from build123d import *

# Parameters (mm, degrees)
SZKIC1_R                         = 11.955497861
SZKIC1_R_2                       = 8
DODANIE_WYCI_GNI_CIE1_DEPTH      = 10
SZKIC2_W                         = 10
SZKIC2_H                         = 23.910995722
DODANIE_WYCI_GNI_CIE2_DEPTH      = 21
SFAZOWANIE1_SIZE                 = 15
SZKIC4_W                         = 9.112824073
SZKIC4_H                         = 13.669236109
DODANIE_WYCI_GNI_CIE4_DEPTH      = 33
DODANIE_WYCI_GNI_CIE5_DEPTH      = 10
DODANIE_WYCI_GNI_CIE5_DEPTH_BACK = 12
SZKIC5_W                         = 41.411530905
SZKIC5_H                         = 13.669236109
SZKIC6_W                         = 16.08298615
SZKIC6_H                         = 27.20632334
WYTNIJ_WYCI_GNI_CIE1_DEPTH       = 54.798638821
WYTNIJ_WYCI_GNI_CIE2_DEPTH       = 54.798638821


with BuildPart() as part:
    # Szkic1 → Dodanie-wyciągnięcie1 (new body)
    with BuildSketch(Plane(origin=(0, 0, 0), x_dir=(0, 0, -1), z_dir=(1, 0, 0))):
        Circle(SZKIC1_R)
        Circle(SZKIC1_R_2, mode=Mode.SUBTRACT)
    extrude(amount=DODANIE_WYCI_GNI_CIE1_DEPTH)

    # Szkic2 → Dodanie-wyciągnięcie2 (add)
    with BuildSketch(Plane.XY):
        with Locations((5, 0)):
            Rectangle(SZKIC2_W, SZKIC2_H)
    extrude(amount=DODANIE_WYCI_GNI_CIE2_DEPTH)

    # Sfazowanie1
    # the kernel refuses this chamfer: 15 mm, written as the material it takes off along each edge
    with BuildSketch(Plane(origin=(0, -50.53074268, 21), x_dir=(0.9996219169112968, 0, 0.02749587661058632), z_dir=(0, 1, 0))) as sfazowanie1_piece_1:
        Polygon((SFAZOWANIE1_SIZE * 0.999621916911, SFAZOWANIE1_SIZE * 0.0274958766106), (-SFAZOWANIE1_SIZE * 0.0274958766106, SFAZOWANIE1_SIZE * 0.999621916911), (0, 0), align=None)
    extrude(amount=101.06148536, mode=Mode.SUBTRACT)

    # Szkic4 → Dodanie-wyciągnięcie4 (add)
    with BuildSketch(Plane(origin=(-3, 0, 3), x_dir=(0.7071067811865513, 0, 0.7071067811865438), z_dir=(-0.7071067811865438, 0, 0.7071067811865513))):
        with Locations((11.369948619, -0.23897266)):
            Rectangle(SZKIC4_W, SZKIC4_H)
    extrude(amount=DODANIE_WYCI_GNI_CIE4_DEPTH)

    # Szkic5 → Dodanie-wyciągnięcie5 (add, two sides: drawn at the far end of the back side and taken through both)
    with BuildSketch(Plane(origin=(11.261637619, 0, 11.261637619), x_dir=(0.7071067811865438, 0, -0.7071067811865512), z_dir=(0.7071067811865512, 0, 0.7071067811865438)).offset(-DODANIE_WYCI_GNI_CIE5_DEPTH_BACK)):
        with Locations((-16.536875235, -0.23897266)):
            Rectangle(SZKIC5_W, SZKIC5_H)
    extrude(amount=DODANIE_WYCI_GNI_CIE5_DEPTH + DODANIE_WYCI_GNI_CIE5_DEPTH_BACK)

    # Szkic6 → Wytnij-wyciągnięcie1 (cut, through all)
    with BuildSketch(Plane(origin=(0, 6.595645395, 0), x_dir=(1, 0, 0), z_dir=(0, 1, 0))):
        with Locations((18.041493075, -17.707460584)):
            Rectangle(SZKIC6_W, SZKIC6_H)
    extrude(amount=-WYTNIJ_WYCI_GNI_CIE1_DEPTH, mode=Mode.SUBTRACT)

    # Szkic7 → Wytnij-wyciągnięcie2 (cut, through all)
    with BuildSketch(Plane(origin=(0, 6.595645395, 0), x_dir=(1, 0, 0), z_dir=(0, 1, 0))):
        Polygon((-23.770482817, -28.898564741), (9.416159533, -28.898564741), (9.416159533, -47.919361128), (-20.148773981, -47.919361128), align=None)
    extrude(amount=-WYTNIJ_WYCI_GNI_CIE2_DEPTH, mode=Mode.SUBTRACT)


solid = part.part
Model file for the job. Use its own axes, mm. A direction names the side the tool comes from. Coordinates: 2 decimals unless noted, no trailing zeros. Write each loop counter-clockwise with the first axis right and the second up, starting at its lowest first coordinate (ties: lowest second). Pieces come first, ordered by that corner, then holes. Notation, with made-up numbers: (-36, 27) -> (-17, 27) arc R13 cw to (-17, 46) -> close; hole circle Ø8 at (38.5, 22). An arc over 180 degrees is marked (long way). One line per item, written item: value. Start each with the question number.
1) Probe probe 1 along Y at (x, z) = (-17.5, 25); probe 2 along Z at (x, y) = (2, -0.5); probe 3 along Z at (x, y) = (6.5, -2.25). List the from-to ranges inside material, lowest first.
2) Slice it at A-A on y = 0. Write the cut outline in (x, z), then the cut area to 3 significant figures.
3) Slice it at B-B on x = 1.5. Write the cut outline in (y, z).
4) Which spindle directions (+Z, -Z, +X, -X, +Y, -Y) get a long thin tool onto all of the face, cutting with end or side? Do faces 1 (the face through (5, 9, 11)), 2 (the face through (10, 0, 8)), 3 (the face through (-3, -7.074, 21)). Say none if no direction does.
5) Slice it at C-C on y = -3. Write the cut outline in (x, z), then the cut area to 3 significant figures.
6) Flat gauge pins, fed straight in: pin 1 Ø1.5 at (x, z) = (-7, 11) entering from -Y; pin 2 Ø4 at (y, z) = (2, 3) entering from -X; pin 3 Ø18.5 at (x, z) = (-5.5, 21) entering from -Y; pin 4 Ø11.5 at (x, z) = (-7.5, 17) entering from +Y. Where does each tip first touch, or does it go through?
7) Slice it at D-D on z = 8. Write the cut outline in (x, y), then the cut area to 3 significant figures.
8) Pull direction Y, two halves, no side cores. Call faces 4 (the face through (5, 0, 0)), 5 (the face through (5, 0, -8)), 6 (the face through (-3, 6.596, 21)), 7 (the face through (0, 0, 1)): +Y half, -Y half, draft (parallel to the pull), parting line (faces both ways), or undercut.
Answers follow:
1. probe 1: -7.07 to 6.6
1. probe 2: -11.95 to -7.98, 0 to 28.9
1. probe 3: -11.74 to -7.68, 0 to 28.9
2. outline: (-23.35, 28.9) -> (0, 5.55) -> (0, 0) -> (5.55, 0) -> (5.72, -0.17) -> (5.9, 0) -> (10, 0) -> (10, 26.67) -> (7.77, 28.9) -> close; (0, -11.96) -> (10, -11.96) -> (10, -8) -> (0, -8) -> close
2. area: 599 mm2
3. outline: (-11.96, 0) arc R11.96 ccw to (11.96, 0) -> (11.96, 7.5) -> (6.6, 7.5) -> (6.6, 28.9) -> (-7.07, 28.9) -> (-7.07, 7.5) -> (-11.96, 7.5) -> close; hole (-8, 0) arc R8 ccw to (8, 0) -> close
4. face 1: +Z, -X, +Y
4. face 2: +Z, -Z, +X, +Y, -Y
4. face 3: +Z, -X, -Y
5. outline: (-23.35, 28.9) -> (0, 5.55) -> (0, 0) -> (5.55, 0) -> (5.72, -0.17) -> (5.9, 0) -> (10, 0) -> (10, 26.67) -> (7.77, 28.9) -> close; (0, -11.57) -> (10, -11.57) -> (10, -7.42) -> (0, -7.42) -> close
5. area: 601 mm2
6. pin 1: through
6. pin 2: x = 0
6. pin 3: y = -7.07
6. pin 4: y = 6.6
7. outline: (-2.45, -7.07) -> (2, -7.07) -> (2, -11.96) -> (10, -11.96) -> (10, 11.96) -> (2, 11.96) -> (2, 6.6) -> (-2.45, 6.6) -> close
7. area: 252 mm2
8. face 4: undercut
8. face 5: undercut
8. face 6: +Y half
8. face 7: draft
